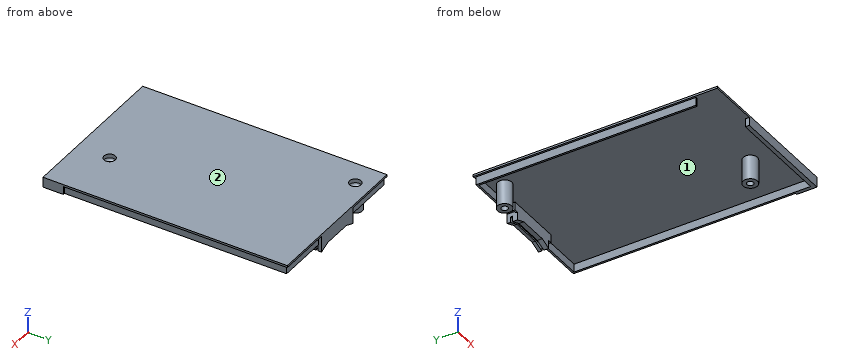
from build123d import *

# Parameters (mm, degrees)
F0_W      = 98.806
F0_H      = 152.4
F1_DEPTH  = 1.27
F3_DEPTH  = 6.35
F4_R      = 4.445
F5_DEPTH  = 15.24
F6_R      = 2.032
F7_DEPTH  = 16.51
F8_R      = 3.556
F9_DEPTH  = 3.81
F11_DEPTH = 6.35
F12_W     = 1.27
F12_H     = 3.556
F13_DEPTH = 30.988
F14_R     = 1.397


with BuildPart() as f1:
    # F0 (on Top) → F1 (new body)
    with BuildSketch(Plane.XY):
        Rectangle(F0_W, F0_H)
    extrude(amount=F1_DEPTH)

    # F2 (on face) → F3 (join)
    with BuildSketch(Plane.XY.offset(1.27)):
        Polygon((-17.653, -73.66), (-17.653, -76.2), (49.403, -76.2), (49.403, -63.5), (48.26, -63.5), (48.26, 75.057), (16.637, 75.057), (16.637, 70.993), (15.494, 70.993), (15.494, 76.2), (-15.494, 76.2), (-15.494, 70.993), (-16.637, 70.993), (-16.637, 75.057), (-48.26, 75.057), (-48.26, -62.23), (-47.117, -62.23), (-47.117, 73.914), (-17.78, 73.914), (-17.78, 69.85), (17.78, 69.85), (17.78, 73.914), (47.117, 73.914), (47.117, -73.66), align=None)
    extrude(amount=-F3_DEPTH)

    # F4 (on face) → F5 (join)
    with BuildSketch(Plane(origin=(0, 0, 0), x_dir=(1, 0, 0), z_dir=(0, 0, -1))):
        with Locations((15.621, 55.88)):
            Circle(F4_R)
        with Locations((-34.163, -66.04)):
            Circle(F4_R)
    extrude(amount=F5_DEPTH)

    # F6 (on face) → F7 (cut, through all)
    with BuildSketch(Plane(origin=(0, 0, -15.24), x_dir=(1, 0, 0), z_dir=(0, 0, -1))):
        with Locations((-34.163, -66.04)):
            Circle(F6_R)
        with Locations((15.621, 55.88)):
            Circle(F6_R)
    extrude(amount=-F7_DEPTH, mode=Mode.SUBTRACT)

    # F8 (on face) → F9 (cut)
    with BuildSketch(Plane.XY.offset(1.27)):
        with Locations((15.621, -55.88)):
            Circle(F8_R)
        with Locations((-34.163, 66.04)):
            Circle(F8_R)
    extrude(amount=-F9_DEPTH, mode=Mode.SUBTRACT)

    # F10 (on face) → F11 (join, through all)
    with BuildSketch(Plane(origin=(0, 76.2, 0), x_dir=(-1, 0, 0), z_dir=(0, 1, 0))):
        Polygon((15.494, -5.08), (-15.494, -5.08), (-15.494, -10.16), (-9.144, -7.62), (9.144, -7.62), (15.494, -10.16), align=None)
    extrude(amount=-F11_DEPTH)

    # F12 (on face) → F13 (cut, through all)
    with BuildSketch(Plane(origin=(-15.494, 0, 0), x_dir=(0, -1, 0), z_dir=(-1, 0, 0))):
        with Locations((-73.533, -8.382)):
            Rectangle(F12_W, F12_H)
    extrude(amount=-F13_DEPTH, mode=Mode.SUBTRACT)

    # F14
    f14_edges = [f1.edges().sort_by_distance(p)[0] for p in [
        (12.065, -55.88, -2.54),
        (-37.719, 66.04, -2.54),
    ]]
    fillet(f14_edges, radius=F14_R)


solid = f1.part
Work out the finished part from the listing and answer in its coordinate system (mm). Face numbers are marked on the shaded views. Coordinates: 2 decimals unless noted, no trailing zeros. Write each loop counter-clockwise with the first axis right and the second up, starting at its lowest first coordinate (ties: lowest second). Pieces come first, ordered by that corner, then holes. Notation, with made-up numbers: M 81,-24.75 L 130,-24.75 A8 ccw 130,-17.75 Z; hole C 40,88 d4. An arc over 180 degrees is marked long. Write item = value, one per line.
1. The part is cut by section D-D (y = 27). Determine the outline of the cut face in (x, z).
Solution:
outline = M -49.4,0 L -48.26,0 L -48.26,-5.08 L -47.12,-5.08 L -47.12,0 L 47.12,0 L 47.12,-5.08 L 48.26,-5.08 L 48.26,0 L 49.4,0 L 49.4,1.27 L -49.4,1.27 Z
2. The part is cut by section A-A (y = -55.88). Determine the outline of the cut face in (x, z) (3 decimals).
Solution:
outline = M -49.403,0 L -48.26,0 L -48.26,-5.08 L -47.117,-5.08 L -47.117,0 L 11.176,0 L 11.176,-15.24 L 13.589,-15.24 L 13.589,-2.54 L 13.462,-2.54 A1.397 cw 12.065,-1.143 L 12.065,1.27 L -49.403,1.27 Z; M 17.653,-15.24 L 20.066,-15.24 L 20.066,0 L 47.117,0 L 47.117,-5.08 L 48.26,-5.08 L 48.26,0 L 49.403,0 L 49.403,1.27 L 19.177,1.27 L 19.177,-1.143 A1.397 cw 17.78,-2.54 L 17.653,-2.54 Z
3. The part is cut by section C-C (z = -13.5). Determine the outline of the cut face in (x, y) (3 decimals).
Solution:
outline = C -34.163,66.04 d8.89; C 15.621,-55.88 d8.89; hole C -34.163,66.04 d4.064; hole C 15.621,-55.88 d4.064
4. The part is cut by section B-B (x = 32.5). Determine the outline of the cut face in (y, z).
Solution:
outline = M -76.2,-5.08 L -73.66,-5.08 L -73.66,0 L 73.91,0 L 73.91,-5.08 L 75.06,-5.08 L 75.06,0 L 76.2,0 L 76.2,1.27 L -76.2,1.27 Z
5. Determine the mould class of the marked faces 1 and 2 for opening direction Y: released by +Y, released by -Y, zero draft, split by the parting line, or undercut.
Solution:
face_1 = undercut
face_2 = zero draft
6. Flat-ended cylindrical pins translate along their axes: pin 1 (8 mm diameter, centred on x = -22, z = -5.5, fed in from +Y); pin 2 (5.5 mm diameter, centred on y = -1, z = -3.5, fed in from -X); pin 3 (1.3 mm diameter, centred on x = -47.5, z = -3.5, fed in from -Y). Find the tip coordinate at first contact, or state that the pin passes through.
Solution:
pin_1 = 75.06
pin_2 = -48.26
pin_3 = -62.23
7. Straight lines are drawn through the part: line 1 (X direction, y = -42.5, z = -4.25); line 2 (X direction, y = 66.04, z = -12.5) (3 decimals); line 3 (X direction, y = -52.5, z = -3). For each, find the intervals that lie inside material, in ascending order. Write a range as from..to.
Solution:
line_1 = -48.26..-47.12, 47.12..48.26
line_2 = -38.608..-36.195, -32.131..-29.718
line_3 = -48.26..-47.12, 12.73..18.51, 47.12..48.26
